Source: three-view drawing plus pictorial views. Frame: mm from the lowest corner of the part. A direction names the side the tool comes from. Coordinates: 2 decimals unless noted, no trailing zeros. Write each loop counter-clockwise with the first axis right and the second up, starting at its lowest first coordinate (ties: lowest second). Pieces come first, ordered by that corner, then holes. Notation, with made-up numbers: (4, -29.5) -> (16, -29.5) arc R28 ccw to (16, -7.5) -> close; hole circle Ø7 at (66, 67.5). An arc over 180 degrees is marked (long way). Write item = value, one per line.
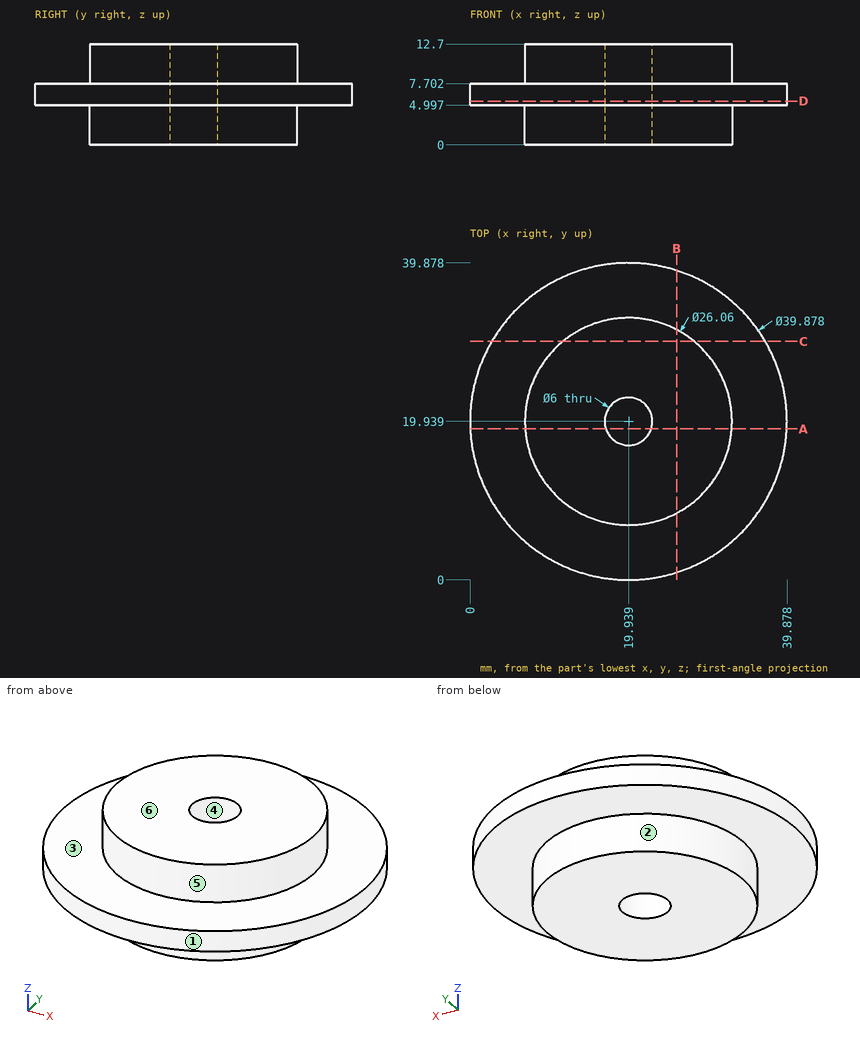
1) Cut plane A-A, the plane y = 19. Output: boundary loops of the cut face in (x, z) (1 decimal).
Answer block:
outline = (0, 5) -> (6.9, 5) -> (6.9, 0) -> (17.1, 0) -> (17.1, 12.7) -> (6.9, 12.7) -> (6.9, 7.7) -> (0, 7.7) -> close; (22.8, 0) -> (32.9, 0) -> (32.9, 5) -> (39.9, 5) -> (39.9, 7.7) -> (32.9, 7.7) -> (32.9, 12.7) -> (22.8, 12.7) -> close
2) Cut plane D-D, the plane z = 5.5. Output: boundary loops of the cut face in (x, y).
Answer block:
outline = circle Ø39.88 at (19.94, 19.94); hole circle Ø6 at (19.94, 19.94)
3) First-contact query: pin 1 Ø3 at (y, z) = (16.5, 1.5) entering from +X; pin 2 Ø1.5 at (x, z) = (12.5, 11) entering from -Y; pin 3 Ø4 at (y, z) = (16, 6) entering from +X. Flat tips, straight axial feed; report the tip coordinate or a pass-through.
Answer block:
pin_1 = 32.82
pin_2 = 8.76
pin_3 = 39.78
4) Reachability of the marked faces 1, 2 and 3 from +Z, -Z, +X, -X, +Y, -Y: full face, straight path, thin tool, end or side. Return the list, or none.
Answer block:
face_1 = +Z, -Z
face_2 = -Z
face_3 = +Z
5) Cut plane C-C, the plane y = 30. Output: boundary loops of the cut face in (x, z) (1 decimal), and give its area (3 significant figures).
Answer block:
outline = (2.7, 5) -> (11.7, 5) -> (11.7, 0) -> (28.2, 0) -> (28.2, 5) -> (37.2, 5) -> (37.2, 7.7) -> (28.2, 7.7) -> (28.2, 12.7) -> (11.7, 12.7) -> (11.7, 7.7) -> (2.7, 7.7) -> close
area = 259 mm2
6) Cut plane B-B, the plane x = 26. Output: boundary loops of the cut face in (y, z) (1 decimal).
Answer block:
outline = (0.9, 5) -> (8.4, 5) -> (8.4, 0) -> (31.5, 0) -> (31.5, 5) -> (38.9, 5) -> (38.9, 7.7) -> (31.5, 7.7) -> (31.5, 12.7) -> (8.4, 12.7) -> (8.4, 7.7) -> (0.9, 7.7) -> close
7) Pull-direction query (X, two-part tool) for the marked faces 4, 5 and 6; classes: +X half, -X half, draft (parallel to the pull), parting line (faces both ways), or undercut.
Answer block:
face_4 = undercut
face_5 = parting line
face_6 = draft
8) Material intervals for probe 1 along Y at (x, z) = (20, 8.75); probe 2 along Z at (x, y) = (4, 15); probe 3 along Y at (x, z) = (24, 2.5), sorted ascending. Write a range as [from, to].
Answer block:
probe_1 = [6.91, 16.94], [22.94, 32.97]
probe_2 = [5, 7.7]
probe_3 = [7.56, 32.32]
